Could you check a few things on this model? Use its own coordinates, in mm. Face numbers are marked on the shaded views. A direction names the side the tool comes from. Round coordinates to 2 decimals unless told otherwise and drop trailing zeros. Write each loop counter-clockwise with the first axis right and the second up, starting at its lowest first coordinate (ties: lowest second). Pieces come first, ordered by that corner, then holes. Notation, with made-up numbers: (53.25, -12.5) -> (88.25, -12.5) arc R23 cw to (88.25, 26.5) -> close; hole circle Ø9 at (55, 6.25). An arc over 180 degrees is marked (long way). Answer in a Markdown table with one row per item.
Autodesk Inventor part; units mm, degrees
ref_plane "YZ Plane" through (0, 0, 0) normal (1, 0, 0) x (0, 1, 0)
ref_plane "XZ Plane" through (0, 0, 0) normal (0, 1, 0) x (-1, 0, 0)
ref_plane "XY Plane" through (0, 0, 0) normal (0, 0, 1) x (1, 0, 0)
sketch "Boceto1" plane through (0, 0, 0) normal (0, 1, 0) x (-1, 0, 0)
  line L0 (0, 0) -> (-3.3, 0)
  line L1 (-3.3, 0) -> (-3.3, -13.3)
  line L2 (-3.3, -13.3) -> (0, -13.3)
  line L3 (0, -13.3) -> (0, 0)
  line L4 (3, 3) -> (-6.3, 3)
  line L5 (-6.3, 3) -> (-6.3, -16.3)
  line L6 (-6.3, -16.3) -> (3, -16.3)
  line L7 (3, -16.3) -> (3, 3)
  dimension "d0" = 3.3
  dimension "d1" = 13.3
  dimension "d2" = 3
extrude "Extrusión1" add sketch "Boceto1" along normal blind 15
fillet "Empalme1" radius 2 4 edges at (6.3, 7.5, 3) (-3, 7.5, 3) (-3, 7.5, -16.3) (6.3, 7.5, -16.3)
sketch "Boceto2" plane through (0, 0, 0) normal (0, -1, 0) x (1, 0, 0)
  line L0 (6.3, 1) -> (6.3, -14.3)
  arc A0 (6.3, 1) -> (4.3, 3) centre (4.3, 1) ccw
  line L1 (-1, 3) -> (4.3, 3)
  arc A1 (-1, 3) -> (-3, 1) centre (-1, 1) ccw
  line L2 (-3, -14.3) -> (-3, 1)
  arc A2 (-3, -14.3) -> (-1, -16.3) centre (-1, -14.3) ccw
  line L3 (4.3, -16.3) -> (-1, -16.3)
  arc A3 (4.3, -16.3) -> (6.3, -14.3) centre (4.3, -14.3) ccw
  point P0 (0, 0)
extrude "Extrusión2" add sketch "Boceto2" along normal blind 3
sketch "Boceto3" plane through (0, 15, 0) normal (0, 1, 0) x (1, 0, 0)
  line L0 (3.3, 13.3) -> (3.3, 0)
  line L1 (6.3, -1) -> (6.3, 14.3)
  line L2 (12.4, -1) -> (12.4, 14.3)
  line L3 (12.4, -1) -> (9.4, -1)
  line L4 (12.4, -1) -> (15.4, -1) construction
  line L5 (9.4, -1) -> (9.4, 2.1)
  line L6 (9.4, 2.1) -> (6.3, 2.1)
  line L7 (12.4, 14.3) -> (9.4, 14.3)
  line L8 (9.4, 14.3) -> (9.4, 11.2)
  line L9 (9.4, 11.2) -> (6.3, 11.2)
  point P0 (0, 0)
  dimension "d8" = 6.1
  dimension "d9" = 3
  dimension "d10" = 180
  dimension "d11" = 3.1
  dimension "d12" = 3.1
extrude "Extrusión3" add sketch "Boceto3" against normal up to surface (18 mm away)
sketch "Boceto4" plane through (0, -3, 0) normal (0, -1, 0) x (1, 0, 0)
  line L0 (3.3, -13.3) -> (3.3, 0)
  line L1 (3.3, 0) -> (0, 0)
  line L2 (0, 0) -> (0, -13.3)
  line L3 (0, -13.3) -> (3.3, -13.3)
  point P0 (1.65, -1.65)
  point P1 (1.65, -11.65)
  point P2 (1.65, -13.3)
  dimension "d15" = 1.65
  dimension "d16" = 1.65
  dimension "d17" = 1.65
hole "Agujero1" at (1.65, -3, -1.65) at (1.65, -3, -11.65) direction (0, 1, 0) diameter 3 end through all
properties part number "cajaIMU"
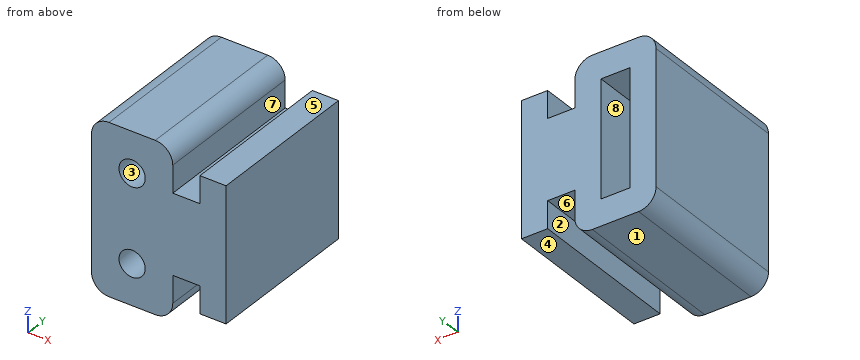
1) Imagine slicing it at C-C, the plane x = 1.65. Please give me the cut outline in (y, z), plus the area to 3 significant figures.
Findings:
| item | result |
|---|---|
| outline | (-3, -16.3) -> (15, -16.3) -> (15, -13.3) -> (0, -13.3) -> (0, -13.15) -> (-3, -13.15) -> close; (-3, -10.15) -> (0, -10.15) -> (0, -3.15) -> (-3, -3.15) -> close; (-3, -0.15) -> (0, -0.15) -> (0, 0) -> (15, 0) -> (15, 3) -> (-3, 3) -> close |
| area | 130 mm^2 |
2) For pin 1 (1.8 mm diameter, centred on x = 1.65, z = -1.65, fed in from +Y); pin 2 (8 mm diameter, centred on x = 8.5, y = 8.5, fed in from +Z); pin 3 (0.9 mm diameter, centred on x = 7.5, y = 5, fed in from -Z); pin 4 (0.9 mm diameter, centred on x = 11.5, y = 9.5, fed in from -Z), each with a flat end and sliding along its axis, tell me the tip position at first contact or that it passes through.
Findings:
| item | result |
|---|---|
| pin 1 | passes through |
| pin 2 | stops at z = 2.99 |
| pin 3 | stops at z = -11.2 |
| pin 4 | stops at z = -14.3 |
3) Imagine slicing it at A-A, the plane z = -11.65. Please give me the cut outline in (x, y).
Findings:
| item | result |
|---|---|
| outline | (-3, -3) -> (0.15, -3) -> (0.15, 0) -> (0, 0) -> (0, 15) -> (-3, 15) -> close; (3.15, -3) -> (6.3, -3) -> (6.3, 15) -> (3.3, 15) -> (3.3, 0) -> (3.15, 0) -> close; (9.4, -3) -> (12.4, -3) -> (12.4, 15) -> (9.4, 15) -> close |
4) For the marked faces 4, 5, 6, 7 and 8, which set-ups out of +Z, -Z, +X, -X, +Y, -Y let a thin tool reach every point of the face, with its end or its side?
Findings:
| item | result |
|---|---|
| face 4 | -Z, +X, +Y, -Y |
| face 5 | +Z, +X, +Y, -Y |
| face 6 | -Z, +Y, -Y |
| face 7 | +Z, +Y, -Y |
| face 8 | +Y |
5) Imagine slicing it at B-B, the plane y = 7.75. Please give me the cut outline in (x, z).
Findings:
| item | result |
|---|---|
| outline | (-3, -14.3) arc R2 ccw to (-1, -16.3) -> (4.3, -16.3) arc R2 ccw to (6.3, -14.3) -> (6.3, -11.2) -> (9.4, -11.2) -> (9.4, -14.3) -> (12.4, -14.3) -> (12.4, 1) -> (9.4, 1) -> (9.4, -2.1) -> (6.3, -2.1) -> (6.3, 1) arc R2 ccw to (4.3, 3) -> (-1, 3) arc R2 ccw to (-3, 1) -> close; hole (0, -13.3) -> (3.3, -13.3) -> (3.3, 0) -> (0, 0) -> close |
6) Imagine slicing it at D-D, the plane z = -7.25. Please give me the cut outline in (x, y), plus the area to 3 significant figures.
Findings:
| item | result |
|---|---|
| outline | (-3, -3) -> (12.4, -3) -> (12.4, 15) -> (3.3, 15) -> (3.3, 0) -> (0, 0) -> (0, 15) -> (-3, 15) -> close |
| area | 228 mm^2 |
7) Please list where these lines run through material, in increasing order: line 1 (Z direction, x = 1.65, y = -0.7); line 2 (X direction, y = -2.15, z = -11.65); line 3 (X direction, y = 4.75, z = -2.5).
Findings:
| item | result |
|---|---|
| line 1 | z = -16.3 to -13.15, -10.15 to -3.15, -0.15 to 3 |
| line 2 | x = -3 to 0.15, 3.15 to 6.3, 9.4 to 12.4 |
| line 3 | x = -3 to 0, 3.3 to 12.4 |
8) Thinking about a two-plate mould opening in Z: for the marked faces 1, 2 and 3, which applies, +Z half, -Z half, draft (parallel to the pull), parting line (faces both ways), or undercut?
Findings:
| item | result |
|---|---|
| face 1 | -Z half |
| face 2 | draft |
| face 3 | undercut |
